Part print with two shaded views. Sizes in mm from the minimum x, y, z corner. Coordinates: 2 decimals unless noted, no trailing zeros. Order: outer loops, then holes, each group sorted by start corner. A loop starts at its lowest first (then second) coordinate and runs counter-clockwise, first axis right, second up.
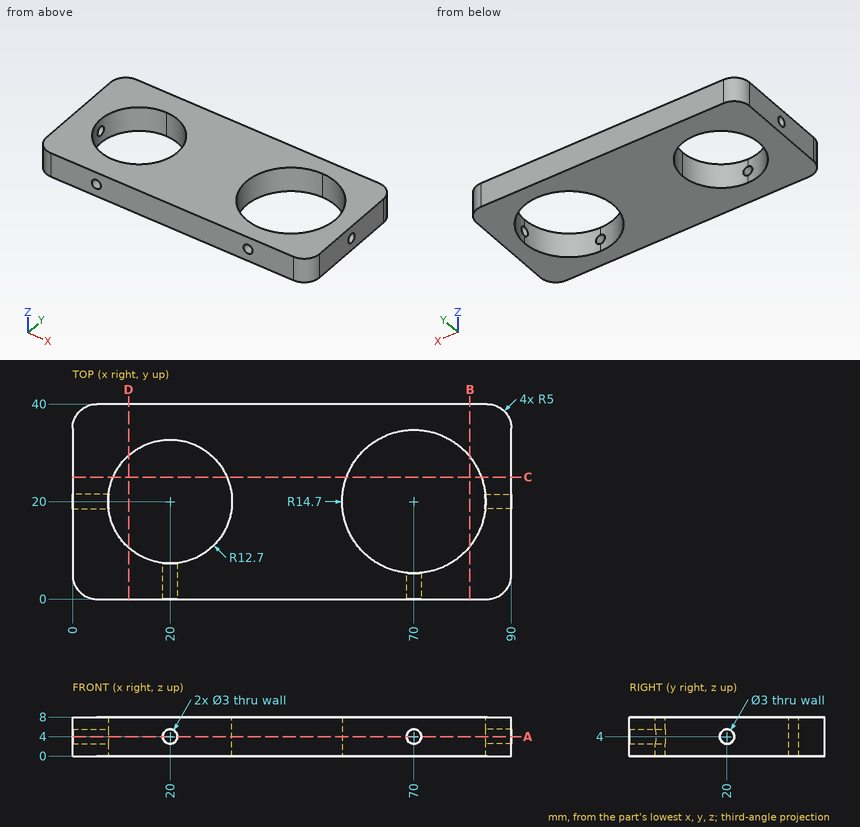
Q1. Cut at B-B on x = 81.5. Write the cut outline in (y, z).
Results list:
outline: (0, 0) - (10.84, 0) - (10.84, 8) - (0, 8) - close; (29.16, 0) - (40, 0) - (40, 8) - (29.16, 8) - close
Q2. Pin check, flat tips, straight feed: pin 1 Ø1.8 at (y, z) = (20, 4) entering from +X; pin 2 Ø2.5 at (x, z) = (20, 4) entering from -Y. Stop position of each tip, or through.
Results list:
pin 1: stops at x = 55.33
pin 2: stops at y = 32.64
Q3. Cut at D-D on x = 11.5. Write the cut outline in (y, z).
Results list:
outline: (0, 0) - (10.56, 0) - (10.56, 8) - (0, 8) - close; (29.44, 0) - (40, 0) - (40, 8) - (29.44, 8) - close
Q4. Cut at A-A on z = 4. Write the cut outline in (x, y).
Results list:
outline: (0, 5) arc R5 ccw to (5, 0) - (18.5, 0) - (18.5, 7.39) arc R12.7 cw to (7.39, 18.5) - (0, 18.5) - close; (0, 21.5) - (7.39, 21.5) arc R12.7 cw (long way) to (21.5, 7.39) - (21.5, 0) - (68.5, 0) - (68.5, 5.38) arc R14.7 cw (long way) to (84.62, 21.5) - (90, 21.5) - (90, 35) arc R5 ccw to (85, 40) - (5, 40) arc R5 ccw to (0, 35) - close; (71.5, 0) - (85, 0) arc R5 ccw to (90, 5) - (90, 18.5) - (84.62, 18.5) arc R14.7 cw to (71.5, 5.38) - close
Q5. Wall check: line 1 along Z through (x, y) = (87.45, 20); line 2 along X through (y, z) = (10, 5.5); line 3 along X through (y, z) = (22.5, 7.5). Give the ranges that are in metal, low to high.
Results list:
line 1: z = 0 to 2.5, 5.5 to 8
line 2: x = 0 to 12.17, 27.83 to 59.23, 80.77 to 90
line 3: x = 0 to 7.55, 32.45 to 55.51, 84.49 to 90
Q6. Cut at C-C on y = 25. Write the cut outline in (x, z), and give its area (3 significant figures).
Results list:
outline: (0, 0) - (8.33, 0) - (8.33, 8) - (0, 8) - close; (31.67, 0) - (56.18, 0) - (56.18, 8) - (31.67, 8) - close; (83.82, 0) - (90, 0) - (90, 8) - (83.82, 8) - close
area: 312 mm2
